Can you work these out from the model? Positions are in its coordinate system, mm. A direction names the side the tool comes from. Round coordinates to 2 decimals unless told otherwise and drop trailing zeros. Order: outer loops, then holes, each group sorted by start corner. A loop starts at its lowest first (then second) coordinate and runs counter-clockwise, first axis right, second up. Notation, with made-up numbers: M -33,-36 L -25,-36 A20 ccw -25,-14 Z; hole C -37.5,48.5 d9. An arc over 180 degrees is marked long. Answer as a JSON object with one key per item and string values. Group by question number.
from build123d import *

# Parameters (mm, degrees)
ESBO_O1_R                = 40
RESSALTO_EXTRUS_O1_DEPTH = 1
CORTE_EXTRUS_O1_START    = -10
CORTE_EXTRUS_O1_DEPTH    = 10
ESBO_O3_R                = 3.5
RESSALTO_EXTRUS_O2_DEPTH = 2
ESBO_O4_R                = 2.5
CORTE_EXTRUS_O2_DEPTH    = 2.5
CHANFRO1_SIZE            = 2
CORTE_EXTRUS_O3_DEPTH    = 3
FILETE1_R                = 4
ESBO_O6_R                = 1.1
CORTE_EXTRUS_O4_DEPTH    = 3
FILETE2_R                = 4
FILETE3_R                = 4
FILETE4_R                = 4
FILETE5_R                = 4
FILETE6_R                = 4
FILETE7_R                = 4
FILETE8_R                = 4
FILETE9_R                = 4
FILETE10_R               = 4
FILETE11_R               = 20


with BuildPart() as part:
    # Esboço1 → Ressalto-extrusão1 (new body)
    with BuildSketch(Plane(origin=(0, 0, 0), x_dir=(1, 0, 0), z_dir=(0, 1, 0))):
        with Locations(Location((0, 0, 0), (0, 0, 270))):
            Circle(ESBO_O1_R)
    extrude(amount=RESSALTO_EXTRUS_O1_DEPTH)

    # Esboço2 → Corte-extrusão1 (cut)
    with BuildSketch(Plane(origin=(0, 1, 0), x_dir=(1, 0, 0), z_dir=(0, 1, 0)).offset(CORTE_EXTRUS_O1_START)):
        with BuildLine():
            ThreePointArc((25, 3), (22, 0), (25, -3))
            Line((25, -3), (39.560670745, -5.912134149))
            ThreePointArc((39.560670745, -5.912134149), (40, 0), (39.560670745, 5.912134149))
            Line((39.560670745, 5.912134149), (25, 3))
        make_face()
        with BuildLine():
            ThreePointArc((-39.560670745, 5.912134149), (-40, 0), (-39.560670745, -5.912134149))
            Line((-39.560670745, -5.912134149), (-25, -3))
            ThreePointArc((-25, -3), (-22, 0), (-25, 3))
            Line((-25, 3), (-39.560670745, 5.912134149))
        make_face()
        with BuildLine():
            Line((9.901923789, -23.150635095), (14.660277009, -37.216612931))
            ThreePointArc((14.660277009, -37.216612931), (20, -34.641016151), (24.900393736, -31.304478782))
            Line((24.900393736, -31.304478782), (15.098076211, -20.150635095))
            ThreePointArc((15.098076211, -20.150635095), (11, -19.052558883), (9.901923789, -23.150635095))
        make_face()
        with BuildLine():
            ThreePointArc((-24.900393736, -31.304478782), (-20, -34.641016151), (-14.660277009, -37.216612931))
            Line((-14.660277009, -37.216612931), (-9.901923789, -23.150635095))
            ThreePointArc((-9.901923789, -23.150635095), (-11, -19.052558883), (-15.098076211, -20.150635095))
            Line((-15.098076211, -20.150635095), (-24.900393736, -31.304478782))
        make_face()
    extrude(amount=CORTE_EXTRUS_O1_DEPTH, mode=Mode.SUBTRACT)

    # Esboço3 → Ressalto-extrusão2 (add)
    with BuildSketch(Plane(origin=(0, 1, 0), x_dir=(1, 0, 0), z_dir=(0, 1, 0))):
        with Locations(Location((0, 0, 0), (0, 0, 270))):
            Circle(ESBO_O3_R)
    extrude(amount=RESSALTO_EXTRUS_O2_DEPTH)

    # Esboço4 → Corte-extrusão2 (cut)
    with BuildSketch(Plane(origin=(0, 3, 0), x_dir=(1, 0, 0), z_dir=(0, 1, 0))):
        with Locations(Location((0, 0, 0), (0, 0, 270))):
            Circle(ESBO_O4_R)
    extrude(amount=-CORTE_EXTRUS_O2_DEPTH, mode=Mode.SUBTRACT)

    # Chanfro1
    chanfro1_edges = [part.edges().sort_by_distance(p)[0] for p in [
        (0, 1, -3.5),
    ]]
    chamfer(chanfro1_edges, length=CHANFRO1_SIZE - 0.0001)  # a hair under: the kernel refuses the full size

    # Esboço5 → Corte-extrusão3 (cut)
    with BuildSketch(Plane(origin=(0, 1, 0), x_dir=(1, 0, 0), z_dir=(0, 1, 0))):
        Polygon((-36.862262331, 15.52976548), (0, 9.495011624), (36.862262331, 15.52976548), (36.862262331, 44.423786918), (-36.862262331, 44.423786918), align=None)
    extrude(amount=-CORTE_EXTRUS_O3_DEPTH, mode=Mode.SUBTRACT)

    # Filete1
    filete1_edges = [part.edges().sort_by_distance(p)[0] for p in [
        (36.862262331, 0.5, -15.52976548),
    ]]
    fillet(filete1_edges, radius=FILETE1_R)

    # Esboço6 → Corte-extrusão4 (cut)
    with BuildSketch(Plane(origin=(0, 0.5, 0), x_dir=(1, 0, 0), z_dir=(0, 1, 0))):
        with Locations(Location((0, 0, 0), (0, 0, 270))):
            Circle(ESBO_O6_R)
    extrude(amount=-CORTE_EXTRUS_O4_DEPTH, mode=Mode.SUBTRACT)

    # Filete2
    filete2_edges = [part.edges().sort_by_distance(p)[0] for p in [
        (-36.862262331, 0.5, -15.52976548),
    ]]
    fillet(filete2_edges, radius=FILETE2_R)

    # Filete3
    filete3_edges = [part.edges().sort_by_distance(p)[0] for p in [
        (-39.560670745, 0.5, -5.912134149),
    ]]
    fillet(filete3_edges, radius=FILETE3_R)

    # Filete4
    filete4_edges = [part.edges().sort_by_distance(p)[0] for p in [
        (-39.560670745, 0.5, 5.912134149),
    ]]
    fillet(filete4_edges, radius=FILETE4_R)

    # Filete5
    filete5_edges = [part.edges().sort_by_distance(p)[0] for p in [
        (-24.900393736, 0.5, 31.304478782),
    ]]
    fillet(filete5_edges, radius=FILETE5_R)

    # Filete6
    filete6_edges = [part.edges().sort_by_distance(p)[0] for p in [
        (-14.660277009, 0.5, 37.216612931),
    ]]
    fillet(filete6_edges, radius=FILETE6_R)

    # Filete7
    filete7_edges = [part.edges().sort_by_distance(p)[0] for p in [
        (14.660277009, 0.5, 37.216612931),
    ]]
    fillet(filete7_edges, radius=FILETE7_R)

    # Filete8
    filete8_edges = [part.edges().sort_by_distance(p)[0] for p in [
        (24.900393736, 0.5, 31.304478782),
    ]]
    fillet(filete8_edges, radius=FILETE8_R)

    # Filete9
    filete9_edges = [part.edges().sort_by_distance(p)[0] for p in [
        (39.560670745, 0.5, 5.912134149),
    ]]
    fillet(filete9_edges, radius=FILETE9_R)

    # Filete10
    filete10_edges = [part.edges().sort_by_distance(p)[0] for p in [
        (39.560670745, 0.5, -5.912134149),
    ]]
    fillet(filete10_edges, radius=FILETE10_R)

    # Filete11
    filete11_edges = [part.edges().sort_by_distance(p)[0] for p in [
        (0, 0.5, -9.495011624),
    ]]
    fillet(filete11_edges, radius=FILETE11_R)


solid = part.part
Item 1: Suppose I cut it at C-C, the plane y = 1.7. Write out the boundary of the cut face in (x, z), and give its area (3 significant figures).
Item 2: If we mould it in two halves opening along Z, with no side actions, what happens to faces 1 (the face through (-1, 0.5, 1)), 2 (the face through (-18.636, 0.507, -12.546)), 3 (the face through (34.565, 0.493, 20.131))? For each: +Z half, -Z half, draft (parallel to the pull), parting line (faces both ways), or undercut.
Item 3: Suppose I cut it at B-B, the plane x = 12.5. Write out the boundary of the cut face in (y, z).
Item 4: Suppose I cut it at D-D, the plane x = 27. Write out the boundary of the cut face in (y, z), and give its area (3 significant figures).
Item 5: I need wall thicknesses on line 1 (X direction, y = 0.2, z = 0); line 2 (Z direction, x = -25, y = 0.65); line 3 (Y direction, x = -21, z = 9). Which ranges of each line are inside material? Lowest first, please.
Item 6: I'm going to push a flat-ended pin straight in: pin 1 Ø1.5 at (x, z) = (22, 0.5) entering from +Y. Where does the tip first touch, or does it pass through?
Item 7: On a 3-axis mill with a long thin cutter (end or side, diameter ignored), from which of +Z, -Z, +X, -X, +Y, -Y can I reach the whole of each face in a straight line? I mean faces 4 (the face through (30.39, 0.49, -4.08)), 5 (the face through (-2.44, 1.77, -0.54)), 6 (the face through (11.614, 0.493, 28.213)), 7 (the face through (-30.24, 0.49, -4.05)). Say none if no direction works.
Computed:
{
 "1": {"outline": "C 0,0 d9.6; hole C 0,0 d5", "area": "52.7 mm^2"},
 "2": {"face 1": "undercut", "face 2": "-Z half", "face 3": "+Z half"},
 "3": {"outline": "M 0,-11.54 L 1,-11.54 L 1,18.65 L 0,18.65 Z; M 0,30.83 L 1,30.83 L 1,37.44 L 0,37.44 Z"},
 "4": {"outline": "M 0,-13.92 L 1,-13.92 L 1,-3.4 L 0,-3.4 Z; M 0,3.4 L 1,3.4 L 1,29.25 L 0,29.25 Z", "area": "36.4 mm^2"},
 "5": {"line 1": "x = -22 to -1.1, 1.1 to 22", "line 2": "z = -13.59 to -3, 3 to 29.64", "line 3": "y = 0 to 1"},
 "6": {"pin 1": "stops at y = 1"},
 "7": {"face 4": "+X, +Y, -Y", "face 5": "+Y", "face 6": "+Y, -Y", "face 7": "-X, +Y, -Y"}
}
